Verification items for the finished model (mm, model axes). Face numbers are marked on the shaded views. Coordinates: 2 decimals unless noted, no trailing zeros. Write each loop counter-clockwise with the first axis right and the second up, starting at its lowest first coordinate (ties: lowest second). Pieces come first, ordered by that corner, then holes. Notation, with made-up numbers: (25, -12.5) -> (29, -12.5) arc R23 cw to (29, 2.5) -> close; hole circle Ø8 at (-36, -15.5). An arc over 180 degrees is marked (long way). Answer in a Markdown table with one row per item.
```python
from build123d import *

# Parameters (mm, degrees)
F1_FACE_R = 32.340866
F2_DEPTH  = 4


with BuildPart() as f1:
    # F0 (on Front) → F1 (revolve)
    with BuildSketch(Plane.XZ):
        Polygon((-13.979599, 18.569916), (-40.269591, 0), (0, 0), (0, 69.063395), (-32.340866, 69.063395), (-13.979599, 54.875147), align=None)
    revolve(axis=Axis((0, 0, 34.531698), (0, 0, -1)))

    # F1_face (on face) → F2 (join)
    with BuildSketch(Plane.XY.offset(69.063395)):
        Circle(F1_FACE_R)
    extrude(amount=-F2_DEPTH)


solid = f1.part
```
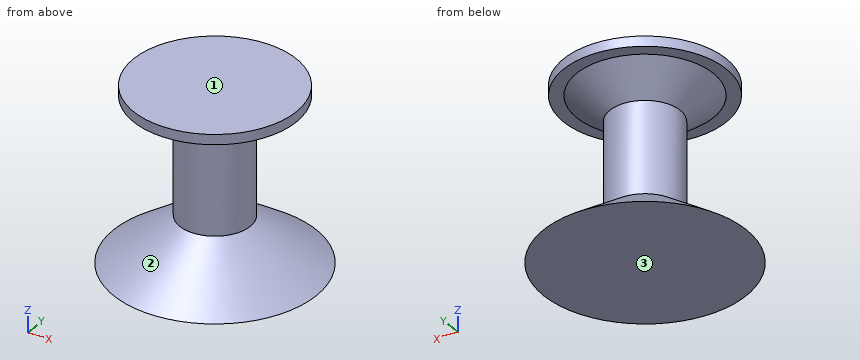
1. Sectioned sample at A-A, the plane y = 0. Record the cut outline in (x, z), and give its area (3 significant figures).
Findings below:
| item | result |
|---|---|
| outline | (-40.27, 0) -> (40.27, 0) -> (13.98, 18.57) -> (13.98, 54.88) -> (27.16, 65.06) -> (32.34, 65.06) -> (32.34, 69.06) -> (-32.34, 69.06) -> (-32.34, 65.06) -> (-27.16, 65.06) -> (-13.98, 54.88) -> (-13.98, 18.57) -> close |
| area | 2,700 mm² |
2. Sectioned sample at C-C, the plane z = 21. Record the cut outline in (x, y).
Findings below:
| item | result |
|---|---|
| outline | circle Ø27.96 at (0, 0) |
3. Release check for a two-part mould opening along Z. For the marked faces 1, 2 and 3 record: released by +Z, released by -Z, zero draft, split by the parting line, or undercut.
Findings below:
| item | result |
|---|---|
| face 1 | released by +Z |
| face 2 | undercut |
| face 3 | released by -Z |
4. Go/stop test with flat-tipped pins: pin 1 (3 mm diameter, centred on x = 6, z = 53, fed in from +Y); pin 2 (10 mm diameter, centred on y = 22.5, z = 14, fed in from -X); pin 3 (5 mm diameter, centred on x = 15, z = 25, fed in from -Y); pin 4 (1.5 mm diameter, centred on x = -20, y = 4.5, fed in from -Z). Record where each tip stops, or that it passes through.
Findings below:
| item | result |
|---|---|
| pin 1 | stops at y = 13.24 |
| pin 2 | stops at x = -17.51 |
| pin 3 | stops at y = -6.26 |
| pin 4 | stops at z = 0 |
5. Material ranges on probe 1 along Z at (x, y) = (20, 22); probe 2 along Z at (x, y) = (-17, 25); probe 3 along Y at (x, z) = (3.5, 16), recorded low to high. Write a range as from..to.
Findings below:
| item | result |
|---|---|
| probe 1 | z = 0..7.44, 65.06..69.06 |
| probe 2 | z = 0..7.09, 65.06..69.06 |
| probe 3 | y = -17.27..17.27 |
